Source: CAD feature listing. Evaluate the final solid. Frame: model axes, mm. Face numbers are marked on the shaded views. A direction names the side the tool comes from. Round coordinates to 2 decimals unless told otherwise and drop trailing zeros. Write each loop counter-clockwise with the first axis right and the second up, starting at its lowest first coordinate (ties: lowest second). Pieces come first, ordered by that corner, then holes.
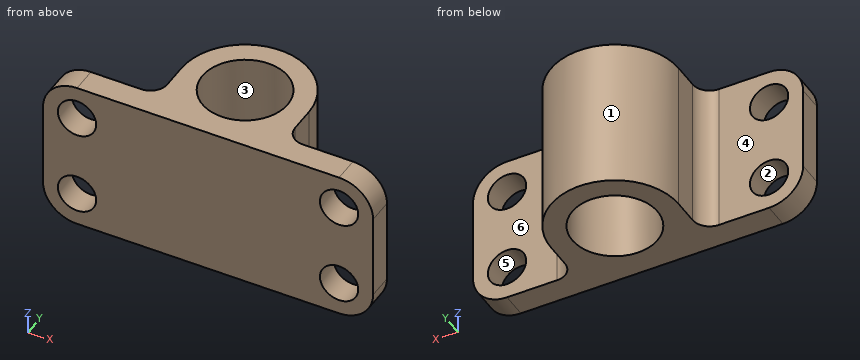
Autodesk Inventor part; units mm, degrees
ref_plane "YZ Plane" through (0, 0, 0) normal (1, 0, 0) x (0, 1, 0)
ref_plane "XZ Plane" through (0, 0, 0) normal (0, 1, 0) x (-1, 0, 0)
ref_plane "XY Plane" through (0, 0, 0) normal (0, 0, 1) x (1, 0, 0)
sketch "スケッチ1" plane through (0, 0, 0) normal (0, 0, 1) x (1, 0, 0)
  line L0 (-19.4, -1.5) -> (19.4, -1.5)
  line L1 (19.4, -1.5) -> (19.4, 1.5)
  line L2 (19.4, 1.5) -> (-19.4, 1.5)
  line L3 (-19.4, 1.5) -> (-19.4, -1.5)
  line L4 (-19.4, -1.5) -> (19.4, 1.5) construction
  line L5 (19.4, -1.5) -> (-19.4, 1.5) construction
  circle A0 centre (0, 6.5) radius 5
  circle A1 centre (0, 6.5) radius 7.5
  line L6 (-7.5, 6.5) -> (-7.5, 1.5)
  line L7 (7.5, 6.5) -> (7.5, 1.5)
  point P0 (0, 0)
  point P1 (0, 0)
  point P2 (0, 0)
  point P3 (0, 0)
  dimension "d4" = 10
  dimension "d5" = 3
  dimension "d6" = 38.8
  dimension "d21" = 15
extrude "押し出し1" add sketch "スケッチ1" along normal mid plane 18
fillet "フィレット1" radius 2 2 edges at (7.5, 1.5, 0) (-7.5, 1.5, 0)
sketch "スケッチ2" plane through (-19.4, -1.5, 9) normal (0, -1, 0) x (1, 0, 0)
  line L0 (4, -14) -> (34.8, -14)
  line L1 (34.8, -14) -> (34.8, -4)
  line L2 (34.8, -4) -> (4, -4)
  line L3 (4, -4) -> (4, -14)
  line L4 (4, -14) -> (34.8, -4) construction
  line L5 (34.8, -14) -> (4, -4) construction
  point P0 (19.4, -9)
  dimension "d11" = 30.8
  dimension "d12" = 10
hole "穴1" at (15.4, -1.5, 5) at (15.4, -1.5, -5) at (-15.4, -1.5, 5) at (-15.4, -1.5, -5) direction (0, 1, 0) diameter 4.5 end through all
fillet "フィレット2" radius 4 4 edges at (-19.4, 0, -9) (-19.4, 0, 9) (19.4, 0, -9) (19.4, 0, 9)
ref_plane "作業平面2" through (0, -1.5, 5) normal (-1, 0, 0) x (0, 0, 1)
ref_plane "作業平面1" through (9.5, 0, 9) normal (0, 1, 0) x (1, 0, 0)
properties part number "scara-base26"
1) Pull-direction query (Y, two-part tool) for the marked faces 1, 2 and 3; classes: released by +Y, released by -Y, zero draft, split by the parting line, or undercut.
Taken from the geometry:
face 1: released by +Y
face 2: zero draft
face 3: undercut
2) Section query D-D on x = 16. Return the cut outline in (y, z).
Taken from the geometry:
outline: (-1.5, -8.95) - (1.5, -8.95) - (1.5, -7.17) - (-1.5, -7.17) - close; (-1.5, -2.83) - (1.5, -2.83) - (1.5, 2.83) - (-1.5, 2.83) - close; (-1.5, 7.17) - (1.5, 7.17) - (1.5, 8.95) - (-1.5, 8.95) - close
3) Contact query for flat-ended pins moving along their axis: P1, Ø2.5, axis at x = -15.4, z = 5, coming from the +Y side; P2, Ø1.5, axis at y = 2.5, z = 2, coming from the +X side; P3, Ø1.5, axis at y = 5, z = -1, coming from the -X side; P4, Ø1, axis at y = 8.5, z = 0.5, coming from the +X side. Output: stop coordinate, or through.
Taken from the geometry:
P1: passes through
P2: stops at x = 8.53
P3: stops at x = -7.5
P4: stops at x = 7.35
4) Section query B-B on z = 1.5. Return the cut outline in (x, y).
Taken from the geometry:
outline: (-19.4, -1.5) - (19.4, -1.5) - (19.4, 1.5) - (9.5, 1.5) arc R2 cw to (7.5, 3.5) - (7.5, 6.5) arc R7.5 ccw to (-7.5, 6.5) - (-7.5, 3.5) arc R2 cw to (-9.5, 1.5) - (-19.4, 1.5) - close; hole circle Ø10 at (0, 6.5)
5) Material intervals for line 1 (X direction, y = 0.15, z = 5); line 2 (Z direction, x = 15.4, y = 0.35); line 3 (X direction, y = 6.5, z = -4.75), sorted ascending.
Taken from the geometry:
line 1: x = -19.4 to -17.65, -13.15 to 13.15, 17.65 to 19.4
line 2: z = -9 to -7.25, -2.75 to 2.75, 7.25 to 9
line 3: x = -7.5 to -5, 5 to 7.5
6) Section query C-C on y = 8.75. Return the cut outline in (x, z).
Taken from the geometry:
outline: (-7.15, -9) - (-4.47, -9) - (-4.47, 9) - (-7.15, 9) - close; (4.47, -9) - (7.15, -9) - (7.15, 9) - (4.47, 9) - close
7) Reachability of the marked faces 4, 5 and 6 from +Z, -Z, +X, -X, +Y, -Y: full face, straight path, thin tool, end or side. Return the list, or none.
Taken from the geometry:
face 4: +Z, -Z, -X, +Y
face 5: +Y, -Y
face 6: +Z, -Z, +X, +Y
8) Section query A-A on y = -0.25. Return the cut outline in (x, z), then the cut area to 3 significant figures.
Taken from the geometry:
outline: (-19.4, -5) arc R4 ccw to (-15.4, -9) - (15.4, -9) arc R4 ccw to (19.4, -5) - (19.4, 5) arc R4 ccw to (15.4, 9) - (-15.4, 9) arc R4 ccw to (-19.4, 5) - close; hole circle Ø4.5 at (-15.4, -5); hole circle Ø4.5 at (-15.4, 5); hole circle Ø4.5 at (15.4, -5); hole circle Ø4.5 at (15.4, 5)
area: 621 mm2
